Geometry: final body of the model. Coordinates: model frame, mm. A direction names the side the tool comes from. Round coordinates to 2 decimals unless told otherwise and drop trailing zeros. Loops run counter-clockwise (first coordinate to the right, second up) from the corner with the lowest first, then second, coordinate; pieces in that order, holes last. Notation, with made-up numbers: (14, 56.25) - (59, 56.25) arc R18 ccw to (59, 71.25) - close; hole circle Ø10 at (26, 54). An arc over 180 degrees is marked (long way). Answer as a JSON object with one key per item and string values. Group by question number.
Item 1: First-contact query: pin 1 (5 mm diameter, centred on x = 2, y = -2, fed in from -Z); pin 2 (2 mm diameter, centred on x = -23.5, y = 13.5, fed in from -Z); pin 3 (1.5 mm diameter, centred on x = 2.5, y = 6.5, fed in from -Z); pin 4 (21 mm diameter, centred on x = 6.5, z = -37, fed in from +Y). Flat tips, straight axial feed; report the tip coordinate or a pass-through.
Item 2: Section A-A (y = 0). Return the cut outline in (x, z).
Item 3: Draft query along X for faces 4 (the face through (-22.5, -4, -14)), 5 (the face through (6.5, 5.08, -1.27)), 6 (the face through (3.96, -22.58, -2.56)), 7 (the face through (-25, -2, -14.8)). Return one class per face: released by +X, released by -X, zero draft, split by the parting line, or undercut.
Item 4: Line query: line 1 (Z direction, x = -4, y = -15); line 2 (Y direction, x = 16, z = -14.5); line 3 (X direction, y = -23.75, z = -35) (3 decimals). Output: solid intervals per line, ascending.
Item 5: Section C-C (z = -20.5). Return the cut outline in (x, y), plus the area to 3 significant figures.
Item 6: Section B-B (x = 14.5). Return the cut outline in (y, z), plus the area to 3 significant figures.
Item 7: Section D-D (z = -32.5). Return the cut outline in (x, y).
Item 8: Reachability of faces 1 (the face through (3.959, -20.789, -4.304)), 2 (the face through (24.76, -23.73, -14.89)), 3 (the face through (-24, 7, -15)) from +Z, -Z, +X, -X, +Y, -Y: full face, straight path, thin tool, end or side. Return the list, or none.
Autodesk Inventor part; units mm, degrees
ref_plane "YZ Plane" through (0, 0, 0) normal (1, 0, 0) x (0, 1, 0)
ref_plane "XZ Plane" through (0, 0, 0) normal (0, 1, 0) x (-1, 0, 0)
ref_plane "XY Plane" through (0, 0, 0) normal (0, 0, 1) x (1, 0, 0)
sketch "Sketch1" plane through (0, 0, 0) normal (0, 0, 1) x (1, 0, 0)
  line L0 (-25, 25) -> (25, 25)
  line L1 (25, 25) -> (25, -25)
  line L2 (25, -25) -> (-25, -25)
  line L3 (-25, -25) -> (-25, 25)
  point P0 (0, 0)
  dimension "d0" = 50
  dimension "d1" = 50
  dimension "d2" = 25
  dimension "d3" = 25
extrude "Extrusion1" add sketch "Sketch1" against normal blind 50
fillet "Fillet1" radius 8.5 3 edges at (0, -25, 0) (-25, 0, 0) (-25, -25, -25)
shell "Shell1" thickness 2.5 removed faces 3 at (-8.3333, 11.1667, -50) at (-8.3333, 25, -36.1667) at (25, 11.1667, -16.6667)
sketch "Sketch2" plane through (-25, -16.5, -8.5) normal (-1, 0, 0) x (0, 0, 1)
  line L0 (0, 41.5) -> (-41.5, 41.5)
  line L1 (-41.5, 41.5) -> (-41.5, 0)
  line L2 (-41.5, 6.5) -> (-6.5, 6.5)
  line L3 (-6.5, 6.5) -> (-6.5, 41.5)
  line L4 (-6.5, 41.5) -> (-41.5, 41.5)
  line L5 (-41.5, 41.5) -> (-41.5, 6.5)
  point P0 (8.5, 16.5)
  dimension "d8" = 35
  dimension "d9" = 35
extrude "Extrusion2" cut sketch "Sketch2" against normal through all
sketch "Sketch3" plane through (-16.5, 25, 0) normal (0, 1, 0) x (1, 0, 0)
  line L0 (41.5, 0) -> (41.5, 2.5)
  line L1 (41.5, 15) -> (11.5, 50)
  line L2 (0, 50) -> (41.5, 50)
  line L3 (41.5, 50) -> (11.5, 50)
  line L4 (41.5, 50) -> (41.5, 15)
  point P0 (41.5, 33)
  point P1 (41.5, 8.5)
  point P2 (16.5, 0)
  point P3 (33, 50)
  point P4 (39, 50)
  dimension "d36" = 30
  dimension "d37" = 35
extrude "Extrusion3" cut sketch "Sketch3" against normal through all
sketch "Sketch4" plane through (0, 0, 0) normal (0, 0, 1) x (1, 0, 0)
  line L0 (-5, -25) -> (25, -25)
  line L1 (-16.5, -25) -> (25, -25)
  line L2 (-16.5, -25) -> (-5, -25)
  line L3 (-25, 25) -> (-25, -10)
  line L4 (-25, 25) -> (-25, -16.5)
  line L5 (-25, -10) -> (-25, -16.5)
  point P0 (0, 0)
  point P1 (2.606, 0)
  dimension "d17" = 27.606
  dimension "d18" = 25
hole "Hole1" at (2.606, 0, 0) direction (0, 0, -1) diameter 12.8 end through all
sketch "Sketch5" plane through (-16.5, -25, -8.5) normal (0, -1, 0) x (1, 0, 0)
  line L0 (12.706, 8.5) -> (25.506, 8.5)
  line L1 (0, 8.5) -> (41.5, 8.5)
  line L2 (41.5, 8.5) -> (0, 8.5)
  line L3 (-8.5, -6.5) -> (-8.5, -41.5)
  point P0 (16.5, 8.5)
  point P1 (12.285, -26.5)
  dimension "d43" = 20.785
  dimension "d44" = 35
hole "Hole2" at (-4.215, -25, -35) direction (0, 1, 0) diameter 8 end through all
sketch "Sketch6" plane through (-16.5, 25, 0) normal (0, 1, 0) x (1, 0, 0)
  arc A0 (-8.5, 8.5) -> (0, 0) centre (0, 8.5) ccw
  line L0 (0, 50) -> (11.5, 50)
  line L1 (-8.5, 15) -> (-8.5, 50)
  line L2 (2, 50) -> (-8.5, 40)
  line L3 (-8.5, 40) -> (-8.5, 50)
  line L4 (-8.5, 50) -> (2, 50)
  point P0 (16.5, 0)
  point P1 (9.6603, 50)
  point P2 (-8.5, 19)
  point P3 (-8.5, 46)
  dimension "d38" = 2
  dimension "d39" = 40
extrude "Extrusion4" cut sketch "Sketch6" against normal through all
fillet "Fillet3" radius 4 7 edges at (-23.75, 25, -15) (-23.75, -10, -41.1905) (-14.5, -23.75, -50) (-5, -23.75, -50) (25, -23.75, -15) (25, 25, -1.25) (-23.75, -10, -15)
equation "\"d0\" = d1"
properties part number "314-06" material "Steel"
Values:
{
 "1": {"pin 1": "passes through", "pin 2": "stops at z = -15", "pin 3": "stops at z = -2.5", "pin 4": "stops at y = -22.5"},
 "2": {"outline": "(-25, -15) - (-22.5, -15) - (-22.5, -8.5) arc R6 cw to (-16.5, -2.5) - (-3.79, -2.5) - (-3.79, 0) - (-16.5, 0) arc R8.5 ccw to (-25, -8.5) - close; (9.01, -2.5) - (25, -2.5) - (25, 0) - (9.01, 0) - close"},
 "3": {"face 4": "released by +X", "face 5": "undercut", "face 6": "zero draft", "face 7": "released by -X"},
 "4": {"line 1": "z = -2.5 to 0", "line 2": "y = -25 to -22.5", "line 3": "x = -20.937 to -8.215, -0.215 to 7.857"},
 "5": {"outline": "(-25, -16.5) arc R8.5 ccw to (-16.5, -25) - (20.29, -25) - (20.29, -22.5) - (-16.5, -22.5) arc R6 cw to (-22.5, -16.5) - (-22.5, -10) - (-25, -10) - close", "area": "137 mm^2"},
 "6": {"outline": "(-25, -27.25) - (-22.5, -27.25) - (-22.5, -8.5) arc R6 cw to (-16.5, -2.5) - (25, -2.5) - (25, 0) - (-16.5, 0) arc R8.5 ccw to (-25, -8.5) - close", "area": "179 mm^2"},
 "7": {"outline": "(-25, -16.5) arc R8.5 ccw to (-16.5, -25) - (-7.34, -25) - (-7.34, -22.5) - (-16.5, -22.5) arc R6 cw to (-22.5, -16.5) - (-22.5, -10) - (-25, -10) - close; (-1.09, -25) - (10, -25) - (10, -22.5) - (-1.09, -22.5) - close"},
 "8": {"face 1": "-Z, +X, +Y", "face 2": "-Z, +X, +Y, -Y", "face 3": "-Z, +X, -X, +Y"}
}
